```python
from build123d import *

# Parameters (mm, degrees)
SKETCH1_W                     = 10.5
SKETCH1_H                     = 5
BASE_DEPTH                    = 3
SKETCH2_W                     = 19
SKETCH2_H                     = 6
FLANGE_DEPTH                  = 0.4
SKETCH3_W                     = 6
SKETCH3_H                     = 3.1
SWITCH_ENCOMPASSING_CUT_DEPTH = 1
SKETCH4_W                     = 3
SKETCH4_H                     = 3
SWITCH_DEPTH                  = 5
SKETCH7_W                     = 7
SKETCH7_H                     = 3
SWITCH_BASE_DEPTH             = 1
SKETCH6_R                     = 0.3
LEG_DEPTH                     = 0.25
L_LEFT_COUNT                  = 2
L_LEFT_PITCH                  = 3.2
L_RIGHT_COUNT                 = 2
L_RIGHT_PITCH                 = 3.2
S_F_R                         = 0.5


with BuildPart() as part:
    # Sketch1 → BASE (new, symmetric)
    with BuildSketch(Plane.XY):
        with Locations((0, 2.5)):
            Rectangle(SKETCH1_W, SKETCH1_H)
    extrude(amount=BASE_DEPTH, both=True)

    # Sketch2 → FLANGE (add)
    with BuildSketch(Plane(origin=(0, 5, 0), x_dir=(1, 0, 0), z_dir=(0, 1, 0))):
        Rectangle(SKETCH2_W, SKETCH2_H)
    extrude(amount=-FLANGE_DEPTH)

    # Sketch3 → SWITCH ENCOMPASSING CUT (cut)
    with BuildSketch(Plane(origin=(0, 5, 0), x_dir=(1, 0, 0), z_dir=(0, 1, 0))):
        Rectangle(SKETCH3_W, SKETCH3_H)
    extrude(amount=-SWITCH_ENCOMPASSING_CUT_DEPTH, mode=Mode.SUBTRACT)

    # Sketch4 → SWITCH (add)
    with BuildSketch(Plane(origin=(0, 4, 0), x_dir=(1, 0, 0), z_dir=(0, 1, 0))):
        with Locations((-1.4, 0)):
            Rectangle(SKETCH4_W, SKETCH4_H)
    extrude(amount=SWITCH_DEPTH)

    # Sketch7 → SWITCH BASE (add)
    with BuildSketch(Plane(origin=(0, 5, 0), x_dir=(1, 0, 0), z_dir=(0, 1, 0))):
        with Locations((-1.4, 0)):
            Rectangle(SKETCH7_W, SKETCH7_H)
    extrude(amount=-SWITCH_BASE_DEPTH)

    # Sketch6 → LEG (add, symmetric)
    with BuildSketch(Plane.XY):
        with BuildLine():
            Line((-0.8, 0), (0.8, 0))
            Line((0.8, 0), (0.8, -2.833030278))
            ThreePointArc((0.8, -2.833030278), (0, -3), (-0.8, -2.833030278))
            Line((-0.8, -2.833030278), (-0.8, 0))
        make_face()
        with Locations((0, -2)):
            Circle(SKETCH6_R, mode=Mode.SUBTRACT)
    leg = extrude(amount=LEG_DEPTH, both=True)

    # L LEFT: LEG ×2
    with Locations(*[(i * L_LEFT_PITCH, 0, 0) for i in range(1, L_LEFT_COUNT)]):
        add(leg)

    # L RIGHT: LEG ×2
    with Locations(*[(-i * L_RIGHT_PITCH, 0, 0) for i in range(1, L_RIGHT_COUNT)]):
        add(leg)

    # S F
    s_f_edges = [part.edges().sort_by_distance(p)[0] for p in [
        (-2.9, 9, 0),
        (0.1, 9, 0),
    ]]
    fillet(s_f_edges, radius=S_F_R)


solid = part.part
```
The model under review builds one solid part; all positions refer to its coordinate system, in mm. A direction names the side the tool comes from. Give positions to 0.01 mm unless a question says otherwise; leave off trailing zeros. Write each loop counter-clockwise with the first axis right and the second up, starting at its lowest first coordinate (ties: lowest second). Pieces come first, ordered by that corner, then holes. Notation, with made-up numbers: (21, 18.5) - (55, 18.5) arc R14 cw to (55, 25.5) - close; hole circle Ø8 at (-38.5, 31). An arc over 180 degrees is marked (long way). Answer in a Markdown table with one row per item. Add a question column.
1. We need section D-D on z = 0.9. Write out the cut boundary in (x, y).
2. We need section A-A on y = -2. Write out the cut boundary in (x, z).
3. Wall thickness on line 1 along Y through (x, z) = (-3.2, 0.1); line 2 along X through (y, z) = (2, -1.45); line 3 along Y through (x, z) = (-1.5, -1.75): over which ranges is each line inside the solid? List them lowest first. Write a range as [from, to].
4. Draft analysis for pull direction X (two halves, no side actions). For faces 5 (the flat face through (5.25, 2, 0)), 6 (the flat face through (-1, 7, 1.5)), 7 (the flat face through (7, 4.6, 0)), state which applies: +X half, -X half, draft (parallel to the pull), parting line (faces both ways), or undercut.
5. Tool access review of faces 1 (the flat face through (-3, -1, 0.25)), 2 (the flat face through (1, 5, 0)), 3 (the flat face through (3, -1, -0.25)), 4 (the flat face through (2.1, 4.5, 0)): name each direction out of +Z, -Z, +X, -X, +Y, -Y from which nothing blocks a thin tool from reaching the whole face with its end or side.
6. We need section C-C on x = 1. Write out the cut boundary in (y, z), then the cut area to 3 significant figures.
7. We need section B-B on x = 3.2. Write out the cut boundary in (y, z), then the cut area to 3 significant figures.
8. Insertion check: P1, Ø1.3, axis at x = -0.5, y = -1, coming from the +Z side; P2, Ø1.5, axis at y = 0, z = 0.5, coming from the +X side; P3, Ø1.3, axis at x = -3.5, y = -1, coming from the -Z side. Each pin has a flat end and moves straight along its axis. Give the tip position at first contact, or say it passes through.
Ans:
| question | item | result |
|---|---|---|
| 1 | outline | (-9.5, 4.6) - (-5.25, 4.6) - (-5.25, 0) - (5.25, 0) - (5.25, 4.6) - (9.5, 4.6) - (9.5, 5) - (3, 5) - (3, 4) - (2.1, 4) - (2.1, 5) - (0.1, 5) - (0.1, 8.5) arc R0.5 ccw to (-0.4, 9) - (-2.4, 9) arc R0.5 ccw to (-2.9, 8.5) - (-2.9, 5) - (-9.5, 5) - close |
| 2 | outline | (-4, -0.25) - (-3.5, -0.25) - (-3.5, 0.25) - (-4, 0.25) - close; (-2.9, -0.25) - (-2.4, -0.25) - (-2.4, 0.25) - (-2.9, 0.25) - close; (-0.8, -0.25) - (-0.3, -0.25) - (-0.3, 0.25) - (-0.8, 0.25) - close; (0.3, -0.25) - (0.8, -0.25) - (0.8, 0.25) - (0.3, 0.25) - close; (2.4, -0.25) - (2.9, -0.25) - (2.9, 0.25) - (2.4, 0.25) - close; (3.5, -0.25) - (4, -0.25) - (4, 0.25) - (3.5, 0.25) - close |
| 3 | line 1 | y = [-3, -2.3], [-1.7, 5] |
| 3 | line 2 | x = [-5.25, 5.25] |
| 3 | line 3 | y = [0, 5] |
| 4 | face 5 | +X half |
| 4 | face 6 | undercut |
| 4 | face 7 | draft |
| 5 | face 1 | +Z, +X, -X, -Y |
| 5 | face 2 | +Z, -Z, +X, +Y |
| 5 | face 3 | -Z, +X, -X, -Y |
| 5 | face 4 | +Y |
| 6 | outline | (0, -3) - (5, -3) - (5, -1.55) - (4, -1.55) - (4, -1.5) - (5, -1.5) - (5, 1.5) - (4, 1.5) - (4, 1.55) - (5, 1.55) - (5, 3) - (0, 3) - close |
| 6 | area | 29.9 mm^2 |
| 7 | outline | (-3, -0.25) - (-2.3, -0.25) - (-2.3, 0.25) - (-3, 0.25) - close; (-1.7, -0.25) - (0, -0.25) - (0, -3) - (5, -3) - (5, 3) - (0, 3) - (0, 0.25) - (-1.7, 0.25) - close |
| 7 | area | 31.2 mm^2 |
| 8 | P1 | stops at z = 0.25 |
| 8 | P2 | stops at x = 5.25 |
| 8 | P3 | stops at z = -0.25 |
